Autodesk Inventor part; units mm, degrees
ref_plane "YZ Plane" through (0, 0, 0) normal (1, 0, 0) x (0, 1, 0)
ref_plane "XZ Plane" through (0, 0, 0) normal (0, 1, 0) x (-1, 0, 0)
ref_plane "XY Plane" through (0, 0, 0) normal (0, 0, 1) x (1, 0, 0)
sketch "Block1" plane through (0, 0, 0) normal (0, 0, 1) x (1, 0, 0)
  circle A0 centre (74.029, 24.2723) radius 1
  line L0 (49.279, 30.4723) -> (71.779, 30.4723)
  line L1 (71.779, 30.4723) -> (71.779, 18.0723)
  line L2 (71.779, 18.0723) -> (49.279, 18.0723)
  line L3 (49.279, 18.0723) -> (49.279, 30.4723)
  line L4 (49.279, 30.4723) -> (44.779, 30.4723)
  line L5 (44.779, 30.4723) -> (44.779, 18.0723)
  line L6 (44.779, 18.0723) -> (49.279, 18.0723)
  line L7 (49.279, 18.0723) -> (49.279, 30.4723)
  line L8 (71.779, 30.4723) -> (76.279, 30.4723)
  line L9 (76.279, 30.4723) -> (76.279, 18.0723)
  line L10 (76.279, 18.0723) -> (71.779, 18.0723)
  line L11 (71.779, 18.0723) -> (71.779, 30.4723)
  line L12 (44.779, 24.2723) -> (76.279, 24.2723) construction
  line L13 (47.029, 30.4723) -> (47.029, 18.0723) construction
  circle A1 centre (47.029, 24.2723) radius 1
  line L14 (74.029, 30.4723) -> (74.029, 18.0723) construction
  point P0 (60.979, 24.0984)
  dimension "d7" = 22.5
  dimension "d8" = 12.4
  dimension "d9" = 4.5
  dimension "d10" = 4.5
  dimension "d11" = 2
  dimension "d12" = 2
sketch "Sketch1" plane through (0, 0, 0) normal (0, 0, 1) x (1, 0, 0)
  line L0 (-92.7646, -8.503) -> (-89.7646, -8.503)
  line L1 (-89.7646, -8.503) -> (-89.7646, -11.753)
  line L2 (-89.7646, -11.753) -> (-92.7646, -11.753)
  line L3 (-92.7646, -11.753) -> (-92.7646, -8.503)
  line L4 (-92.7646, -21.6527) -> (-89.7646, -21.6527)
  line L5 (-89.7646, -21.6527) -> (-89.7646, -21.7527)
  line L6 (-89.7646, -21.7527) -> (-92.7646, -21.7527)
  line L7 (-92.7646, -21.7527) -> (-92.7646, -21.6527)
  line L8 (-7, -8.25) -> (7, -8.25)
  line L9 (7, -8.25) -> (7, -5)
  line L10 (7, -5) -> (-7, -5)
  line L11 (-7, -5) -> (-7, -8.25)
  line L12 (-10, 5) -> (10, 5)
  line L13 (10, 5) -> (10, -5)
  line L14 (10, -5) -> (-10, -5)
  line L15 (-10, -5) -> (-10, 5)
  line L16 (0, -5) -> (0, 5) construction
  line L17 (0, -5) -> (0, -8.25) construction
  line L18 (-10, 0) -> (10, 0) construction
  line L19 (-7, 8.25) -> (7, 8.25)
  line L20 (7, 8.25) -> (7, 5)
  line L21 (7, 5) -> (-7, 5)
  line L22 (-7, 5) -> (-7, 8.25)
  line L23 (0, 5) -> (0, -5) construction
  line L24 (0, 5) -> (0, 8.25) construction
  point P0 (0, 0)
  dimension "d0" = 3
  dimension "mat" = 3.25
  dimension "d2" = 3
  dimension "d3" = 0.1
  dimension "d34" = 14
  dimension "d35" = 3.25
  dimension "d36" = 20
  dimension "d37" = 10
extrude "Extrusion4" add sketch "Sketch1" along normal blind 3.25 contours L11 L10 L9 L8 | L14 L15 L12 L13 L10 | L22 L19 L20 L12
equation "\"d35\" = mat"
equation "\"d38\" = mat"
properties part number "arm-servo"
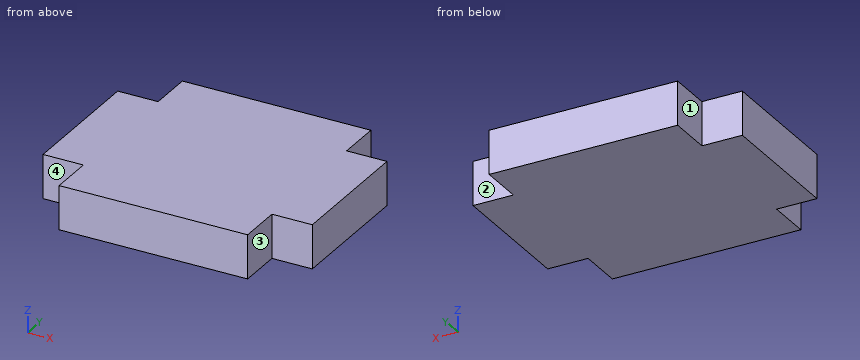
Source: CAD feature listing. Evaluate the final solid. Frame: model axes, mm. Face numbers are marked on the shaded views. A direction names the side the tool comes from. Coordinates: 2 decimals unless noted, no trailing zeros. Loops run counter-clockwise (first coordinate to the right, second up) from the corner with the lowest first, then second, coordinate; pieces in that order, holes last. Notation, with made-up numbers: (70.5, 35.25) - (84.5, 35.25) arc R32 ccw to (84.5, 71.25) - close; hole circle Ø2 at (-15, -0.75). An arc over 180 degrees is marked (long way). Return JSON: item names as keys, results as strings.
Q1. Section B-B, the plane y = 7. Return loops of the section in (x, z), plus the area to 3 significant figures.
Results:
{"outline": "(-7, 0) - (7, 0) - (7, 3.25) - (-7, 3.25) - close", "area": "45.5 mm2"}
Q2. Material intervals for line 1 along X through (y, z) = (6.75, 0.9); line 2 along Y through (x, z) = (8, 0.7), sorted ascending.
Results:
{"line 1": "-7 to 7", "line 2": "-5 to 5"}
Q3. Section C-C, the plane x = -8.25. Return loops of the section in (y, z), plus the area to 3 significant figures.
Results:
{"outline": "(-5, 0) - (5, 0) - (5, 3.25) - (-5, 3.25) - close", "area": "32.5 mm2"}
Q4. Access query for the marked faces 1, 2, 3 and 4. Directions: +Z, -Z, +X, -X, +Y, -Y. A direction counts if a zero-diameter tool reaches every point of the face in a straight line with its end or side. Return the directions, or none.
Results:
{"face 1": "+Z, -Z, -X, +Y", "face 2": "+Z, -Z, +X, +Y", "face 3": "+Z, -Z, +X, -Y", "face 4": "+Z, -Z, -X, -Y"}
Q5. Section A-A, the plane z = 2.7. Return loops of the section in (x, y), plus the area to 3 significant figures.
Results:
{"outline": "(-10, -5) - (-7, -5) - (-7, -8.25) - (7, -8.25) - (7, -5) - (10, -5) - (10, 5) - (7, 5) - (7, 8.25) - (-7, 8.25) - (-7, 5) - (-10, 5) - close", "area": "291 mm2"}
Q6. Contact query for flat-ended pins moving along their axis: P1, Ø1.6, axis at y = -7, z = 1.5, coming from the -X side; P2, Ø1.5, axis at x = -8.5, z = 1.5, coming from the -Y side; P3, Ø0.9, axis at x = 8, z = 1, coming from the +Y side. Output: stop coordinate, or through.
Results:
{"P1": "x = -7", "P2": "y = -5", "P3": "y = 5"}
